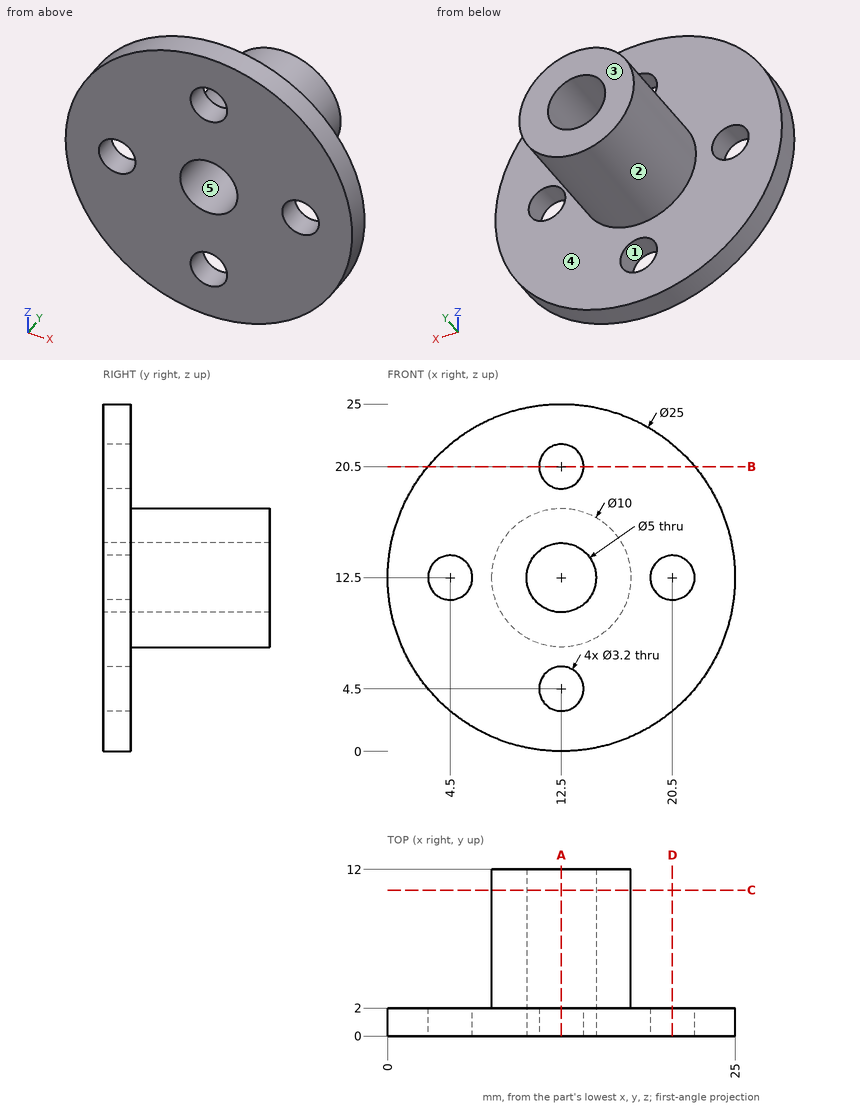
The figure shows three views and two pictorial views of one solid part (mm, origin at its lowest corner). Answer the questions. A direction names the side the tool comes from. Give positions to 0.01 mm unless a question says otherwise; leave off trailing zeros. Write each loop counter-clockwise with the first axis right and the second up, starting at its lowest first coordinate (ties: lowest second). Pieces come first, ordered by that corner, then holes. Notation, with made-up numbers: (30.25, 68) - (66.25, 68) arc R26 ccw to (66.25, 87) - close; hole circle Ø11 at (54, 69). An arc over 180 degrees is marked (long way). Use one line per item in the form item = value. Start each with the question number.
1) Find section A-A on x = 12.5. Determine the outline of the cut face in (y, z).
2) Find section B-B on z = 20.5. Determine the outline of the cut face in (x, y).
3) Flat-ended cylindrical pins translate along their axes: pin 1 Ø6 at (x, z) = (12.5, 12.5) entering from +Y; pin 2 Ø3.5 at (x, z) = (20.5, 12.5) entering from +Y; pin 3 Ø1.5 at (x, y) = (21, 2.5) entering from +Z; pin 4 Ø2 at (x, y) = (16, 6) entering from +Z. Find the tip coordinate at first contact, or state that the pin passes through.
4) A tool of negligible diameter and unlimited length cuts with its end or side. For the marked faces 4 and 5, from which of +Z, -Z, +X, -X, +Y, -Y can it reach the whole face along a straight path? Write none if from no direction.
5) Consider line 1 along Z through (x, y) = (12.5, 1); line 2 along Z through (x, y) = (4.5, 1.65); line 3 along Y through (x, z) = (15.5, 4.25). Determine where each line is inside the solid, lowest interval first. Write a range as from..to.
6) Find section D-D on x = 20.5. Determine the outline of the cut face in (y, z), plus the area to 3 significant figures.
7) Find section C-C on y = 10.5. Determine the outline of the cut face in (x, z).
8) The mould has two halves that part along X. Classify the marked faces 1, 2 and 3: pulls with the +X half, pulls with the -X half, needs draft (parallel to the pull), parting line crosses it, or undercut.
Geometry results:
q1.outline = (0, 0) - (2, 0) - (2, 2.9) - (0, 2.9) - close; (0, 6.1) - (2, 6.1) - (2, 7.5) - (12, 7.5) - (12, 10) - (0, 10) - close; (0, 15) - (12, 15) - (12, 17.5) - (2, 17.5) - (2, 18.9) - (0, 18.9) - close; (0, 22.1) - (2, 22.1) - (2, 25) - (0, 25) - close
q2.outline = (2.9, 0) - (10.9, 0) - (10.9, 2) - (2.9, 2) - close; (14.1, 0) - (22.1, 0) - (22.1, 2) - (14.1, 2) - close
q3.pin_1 = 12
q3.pin_2 = 2
q3.pin_3 = 22.15
q3.pin_4 = 16.83
q4.face_4 = +Y
q4.face_5 = +Y, -Y
q5.line_1 = 0..2.9, 6.1..10, 15..18.9, 22.1..25
q5.line_2 = 2.9..10.9, 14.1..22.1
q5.line_3 = 0..2
q6.outline = (0, 2.9) - (2, 2.9) - (2, 10.9) - (0, 10.9) - close; (0, 14.1) - (2, 14.1) - (2, 22.1) - (0, 22.1) - close
q6.area = 32.0 mm2
q7.outline = circle Ø10 at (12.5, 12.5); hole circle Ø5 at (12.5, 12.5)
q8.face_1 = undercut
q8.face_2 = parting line crosses it
q8.face_3 = needs draft
